Geometry check sheet. Reference: the model listing, model coordinates, mm. Face numbers are marked on the shaded views. Give positions to 0.01 mm unless a question says otherwise; leave off trailing zeros. Write each loop counter-clockwise with the first axis right and the second up, starting at its lowest first coordinate (ties: lowest second). Pieces come first, ordered by that corner, then holes.
(1) Mould release check, pull along Y, two halves, no side actions. Record for the marked faces 1, 2, 3 and 4: +Y half, -Y half, draft (parallel to the pull), parting line (faces both ways), or undercut.
(2) Cross-section at B-B (x = -14.5). Record the boundary of the cut face in (y, z), and give its area (3 significant figures).
(3) Cross-section at C-C (z = 4). Record the boundary of the cut face in (x, y).
(4) Depth check by flat-ended pin: P1, Ø10, axis at x = -24.5, y = 8, coming from the +Z side; P2, Ø23, axis at x = -22.12, y = 6.17, coming from the +Z side. Enter the tip coordinate at first touch or a pass-through.
(5) Thickness scan on line 1 along Y through (x, z) = (-21.5, 5.5); line 2 along X through (y, z) = (12, 7.5); line 3 along X through (y, z) = (10, 19). Record the ranges inside material, lowest first.
(6) Cross-section at A-A (y = 14). Record the boundary of the cut face in (x, z).
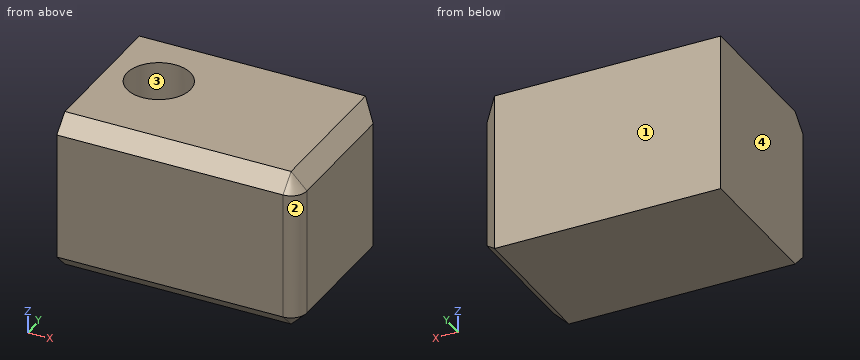
```python
from build123d import *

# Parameters (mm, degrees)
F0_W     = 76.2
F0_H     = 50.8
F1_DEPTH = 25
F2_R     = 10
F3_DEPTH = 25
F4_R     = 5
F5_SIZE  = 5


with BuildPart() as f1:
    # F0 (on Top) → F1 (new body, symmetric)
    with BuildSketch(Plane.XY):
        Rectangle(F0_W, F0_H)
    extrude(amount=F1_DEPTH, both=True)

    # F2 (on face) → F3 (cut)
    with BuildSketch(Plane.XY.offset(25)):
        with Locations((-22.124985, 6.172692)):
            Circle(F2_R)
    extrude(amount=-F3_DEPTH, mode=Mode.SUBTRACT)

    # F4
    f4_edges = [f1.edges().sort_by_distance(p)[0] for p in [
        (38.1, -25.4, 0),
    ]]
    fillet(f4_edges, radius=F4_R)

    # F5
    f5_edges = [f1.edges().sort_by_distance(p)[0] for p in [
        (38.1, 2.5, -25),
        (38.1, -20.4, 0),
        (38.1, 25.4, 0),
        (38.1, 2.5, 25),
    ]]
    chamfer(f5_edges, length=F5_SIZE)


solid = f1.part
```
Reply:
1. face 1: +Y half
1. face 2: -Y half
1. face 3: undercut
1. face 4: draft
2. outline: (-25.4, -20) - (-20.4, -25) - (25.4, -25) - (25.4, 25) - (12.64, 25) - (12.64, 0) - (-0.3, 0) - (-0.3, 25) - (-20.4, 25) - (-25.4, 20) - close
2. area: 2,190 mm2
3. outline: (-38.1, -25.4) - (33.1, -25.4) arc R5 ccw to (38.1, -20.4) - (38.1, 20.4) - (33.1, 25.4) - (-38.1, 25.4) - close; hole circle Ø20 at (-22.12, 6.17)
4. P1: stops at z = 0
4. P2: stops at z = 25
5. line 1: y = -25.4 to -3.81, 16.15 to 25.4
5. line 2: x = -38.1 to -30.25, -14 to 38.1
5. line 3: x = -38.1 to -31.36, -12.89 to 38.1
6. outline: (-38.1, -25) - (33.1, -25) - (38.1, -20) - (38.1, 20) - (33.1, 25) - (-15.9, 25) - (-15.9, 0) - (-28.35, 0) - (-28.35, 25) - (-38.1, 25) - close
